The drawing under review shows one solid part. Ordinate dimensions are in mm from its lowest x, y, z. Coordinates: 2 decimals unless noted, no trailing zeros. Write each loop counter-clockwise with the first axis right and the second up, starting at its lowest first coordinate (ties: lowest second). Pieces come first, ordered by that corner, then holes.
Q1. Add section B-B, the plane y = 2.25. Give the boundary of the cut face in (x, z), plus the area to 3 significant figures.
Q2. To check wall thickness, follow probe 1 along Z at (x, y) = (139.7, 8.5); probe 2 along X at (y, z) = (8.25, 57.5); probe 3 along Z at (x, y) = (134.5, 9.5). State the ranges of each line that lie inside material, in increasing order.
Q3. The part is to be moulded in two halves that separate along Z. For the marked faces 1, 2 and 3, say which applies: +Z half, -Z half, draft (parallel to the pull), parting line (faces both ways), or undercut.
Q4. Add section A-A, the plane x = 139.7. Give the boundary of the cut face in (y, z), plus the area to 3 significant figures.
Q5. Add section C-C, the plane z = 57.15. Give the boundary of the cut face in (x, y), plus the area to 3 significant figures.
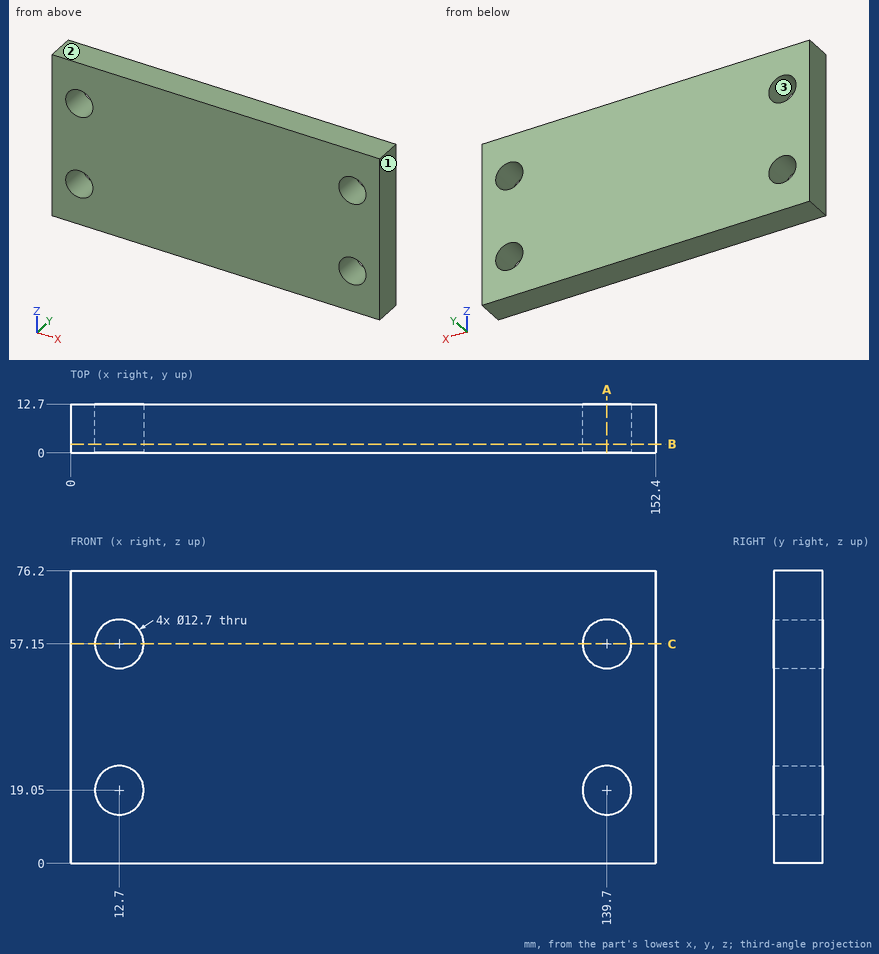
Here are the results:
1. outline: (0, 0) - (152.4, 0) - (152.4, 76.2) - (0, 76.2) - close; hole circle Ø12.7 at (12.7, 19.05); hole circle Ø12.7 at (12.7, 57.15); hole circle Ø12.7 at (139.7, 19.05); hole circle Ø12.7 at (139.7, 57.15)
1. area: 11,100 mm2
2. probe 1: z = 0 to 12.7, 25.4 to 50.8, 63.5 to 76.2
2. probe 2: x = 0 to 6.36, 19.04 to 133.36, 146.04 to 152.4
2. probe 3: z = 0 to 15.41, 22.69 to 53.51, 60.79 to 76.2
3. face 1: draft
3. face 2: +Z half
3. face 3: undercut
4. outline: (0, 0) - (12.7, 0) - (12.7, 12.7) - (0, 12.7) - close; (0, 25.4) - (12.7, 25.4) - (12.7, 50.8) - (0, 50.8) - close; (0, 63.5) - (12.7, 63.5) - (12.7, 76.2) - (0, 76.2) - close
4. area: 645 mm2
5. outline: (0, 0) - (6.35, 0) - (6.35, 12.7) - (0, 12.7) - close; (19.05, 0) - (133.35, 0) - (133.35, 12.7) - (19.05, 12.7) - close; (146.05, 0) - (152.4, 0) - (152.4, 12.7) - (146.05, 12.7) - close
5. area: 1,610 mm2
